Geometry: final body of the model. Coordinates: model frame, mm. Face numbers are marked on the shaded views. A direction names the side the tool comes from. Give positions to 0.01 mm unless a question says otherwise; leave off trailing zeros. Loops run counter-clockwise (first coordinate to the right, second up) from the corner with the lowest first, then second, coordinate; pieces in that order, holes last. Notation, with made-up numbers: (30, -34.5) -> (74, -34.5) arc R13 cw to (74, -14.5) -> close; hole circle Ø5 at (46.5, 69.25). An arc over 180 degrees is marked (long way). Answer in a Markdown table with one row per item. Add a question column.
from build123d import *

# Parameters (mm, degrees)
F0_W     = 50
F0_H     = 5
F1_DEPTH = 3
F2_R     = 0.5
F3_DEPTH = 5
F4_R     = 3.5
F5_DEPTH = 25


with BuildPart() as f1:
    # F0 (on Top) → F1 (new body)
    with BuildSketch(Plane.XY):
        with Locations((25, 2.5)):
            Rectangle(F0_W, F0_H)
    extrude(amount=F1_DEPTH)

    # F2 (on face) → F3 (join)
    with BuildSketch(Plane(origin=(0, 5, 0), x_dir=(-1, 0, 0), z_dir=(0, 1, 0))):
        with Locations((-1.5, 1.5)):
            Circle(F2_R)
    extrude(amount=F3_DEPTH)

    # F4 (on face) → F5 (join)
    with BuildSketch(Plane(origin=(0, 5, 0), x_dir=(-1, 0, 0), z_dir=(0, 1, 0))):
        with Locations((-45, 1.5)):
            Circle(F4_R)
    extrude(amount=F5_DEPTH)


solid = f1.part
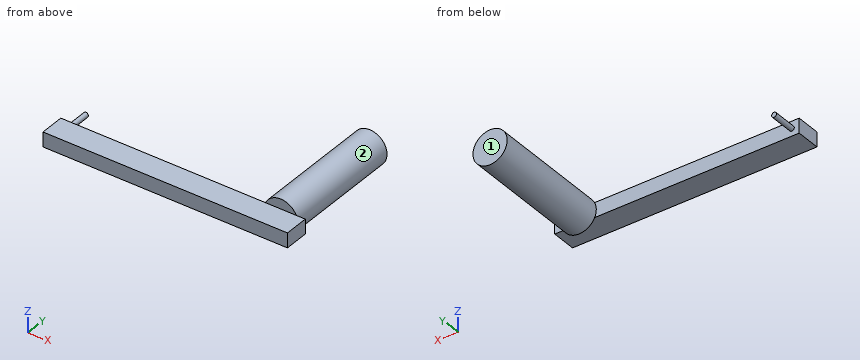
(1) Pin query (flat end, axial travel): pin 1 Ø4 at (y, z) = (3.5, -0.5) entering from -X; pin 2 Ø1 at (y, z) = (6.5, -1) entering from -X; pin 3 Ø2.5 at (x, y) = (19, 3) entering from -Z; pin 4 Ø5.5 at (x, y) = (34, 2) entering from +Z. Return the tip coordinate at first contact, or that it passes through.
(2) Reachability of the marked faces 1 and 2 from +Z, -Z, +X, -X, +Y, -Y: full face, straight path, thin tool, end or side. Return the list, or none.
(3) Cut plane C-C on y = 9. Return the cut outline in (x, z), then the cut area to 3 significant figures.
(4) Material intervals for line 1 along X through (y, z) = (15.75, 3); line 2 along X through (y, z) = (13.75, 1.75); line 3 along Y through (x, z) = (17, 1.5), sorted ascending. Write a range as from..to.
(5) Cut plane D-D on x = 1.5. Return the cut outline in (y, z).
(6) Cut plane A-A on x = 45. Return the cut outline in (y, z).
(7) Cut plane B-B on z = 1.5. Return the cut outline in (x, y).
Answer list:
| question | item | result |
|---|---|---|
| 1 | pin 1 | stops at x = 0 |
| 1 | pin 2 | stops at x = 42.13 |
| 1 | pin 3 | stops at z = 0 |
| 1 | pin 4 | stops at z = 3 |
| 2 | face 1 | +Z, -Z, +X, -X, +Y |
| 2 | face 2 | +Y |
| 3 | outline | circle Ø1 at (1.5, 1.5); circle Ø7 at (45, 1.5) |
| 3 | area | 39.3 mm² |
| 4 | line 1 | x = 41.84..48.16 |
| 4 | line 2 | x = 41.51..48.49 |
| 4 | line 3 | y = 0..5 |
| 5 | outline | (0, 0) -> (5, 0) -> (5, 1) -> (10, 1) -> (10, 2) -> (5, 2) -> (5, 3) -> (0, 3) -> close |
| 6 | outline | (0, 0) -> (5, 0) -> (5, -2) -> (30, -2) -> (30, 5) -> (5, 5) -> (5, 3) -> (0, 3) -> close |
| 7 | outline | (0, 0) -> (50, 0) -> (50, 5) -> (48.5, 5) -> (48.5, 30) -> (41.5, 30) -> (41.5, 5) -> (2, 5) -> (2, 10) -> (1, 10) -> (1, 5) -> (0, 5) -> close |
